Geometry: final body of the model. Coordinates: model frame, mm. Face numbers are marked on the shaded views. A direction names the side the tool comes from. Give positions to 0.01 mm unless a question says otherwise; leave off trailing zeros. Write each loop counter-clockwise with the first axis right and the second up, starting at its lowest first coordinate (ties: lowest second). Pieces come first, ordered by that corner, then holes. Notation, with made-up numbers: M 81.5,-12 L 112.5,-12 A27 ccw 112.5,4 Z; hole C 20.25,36 d2. An arc over 180 degrees is marked long. One line per question, with ' | ' between items.
from build123d import *

# Parameters (mm, degrees)
M3X0_5_TAPPED_HOLE1_D               = 2.5
M3X0_5_TAPPED_HOLE1_DEPTH           = 3.248924226
M3X0_5_TAPPED_HOLE1_TIP             = 0.751075774
BOSS_EXTRUDE1_DEPTH                 = 40
M3X0_5_TAPPED_HOLE2_D               = 2.5
M3X0_5_TAPPED_HOLE2_DEPTH           = 5
M3X0_5_TAPPED_HOLE2_TIP             = 0.751075774
M3X0_5_TAPPED_HOLE2_ON_FACE_2_D     = 2.5
M3X0_5_TAPPED_HOLE2_ON_FACE_2_DEPTH = 5
M3X0_5_TAPPED_HOLE2_ON_FACE_2_TIP   = 0.751075774


with BuildPart() as part:
    # Sketch1 → Revolve1 (revolve)
    with BuildSketch(Plane.XY):
        Polygon((0, 0), (0, 17.5), (10, 17.5), (10, 12.5), (20, 12.5), (20, 17.5), (40, 17.5), (40, 0), align=None)
    revolve(axis=Axis((0, 0, 0), (1, 0, 0)))

    # M3x0.5 Tapped Hole1
    with Locations(Plane(origin=(31.5, 0, 17.5), x_dir=(1, 0, 0), z_dir=(0, 0, 1))):
        with Locations((0, 0)):
            Hole(M3X0_5_TAPPED_HOLE1_D / 2, depth=M3X0_5_TAPPED_HOLE1_DEPTH)
            with Locations((0, 0, -(M3X0_5_TAPPED_HOLE1_DEPTH + M3X0_5_TAPPED_HOLE1_TIP / 2))):  # 118° drill point
                Cone(0, M3X0_5_TAPPED_HOLE1_D / 2, M3X0_5_TAPPED_HOLE1_TIP, mode=Mode.SUBTRACT)

    # Sketch3 → Boss-Extrude1 (add)
    with BuildSketch(Plane(origin=(40, 0, 0), x_dir=(0, 0, -1), z_dir=(1, 0, 0))):
        with BuildLine():
            Line((-12.247448714, -12.5), (-12.247448714, 12.5))
            ThreePointArc((-12.247448714, 12.5), (0, 17.5), (12.247448714, 12.5))
            Line((12.247448714, 12.5), (12.247448714, -12.5))
            ThreePointArc((12.247448714, -12.5), (0, -17.5), (-12.247448714, -12.5))
        make_face()
    extrude(amount=BOSS_EXTRUDE1_DEPTH)

    # M3x0.5 Tapped Hole2
    with Locations(Plane(origin=(50, 0, 12.247448714), x_dir=(1, 0, 0), z_dir=(0, 0, 1))):
        with Locations((0, 0), (15, 0)):
            Hole(M3X0_5_TAPPED_HOLE2_D / 2, depth=M3X0_5_TAPPED_HOLE2_DEPTH)
            with Locations((0, 0, -(M3X0_5_TAPPED_HOLE2_DEPTH + M3X0_5_TAPPED_HOLE2_TIP / 2))):  # 118° drill point
                Cone(0, M3X0_5_TAPPED_HOLE2_D / 2, M3X0_5_TAPPED_HOLE2_TIP, mode=Mode.SUBTRACT)

    # M3x0.5 Tapped Hole2 on face 2
    with Locations(Plane(origin=(65, 0, -12.247448714), x_dir=(-1, 0, 0), z_dir=(0, 0, -1))):
        with Locations((0, 0), (15, 0)):
            Hole(M3X0_5_TAPPED_HOLE2_ON_FACE_2_D / 2, depth=M3X0_5_TAPPED_HOLE2_ON_FACE_2_DEPTH)
            with Locations((0, 0, -(M3X0_5_TAPPED_HOLE2_ON_FACE_2_DEPTH + M3X0_5_TAPPED_HOLE2_ON_FACE_2_TIP / 2))):  # 118° drill point
                Cone(0, M3X0_5_TAPPED_HOLE2_ON_FACE_2_D / 2, M3X0_5_TAPPED_HOLE2_ON_FACE_2_TIP, mode=Mode.SUBTRACT)


solid = part.part
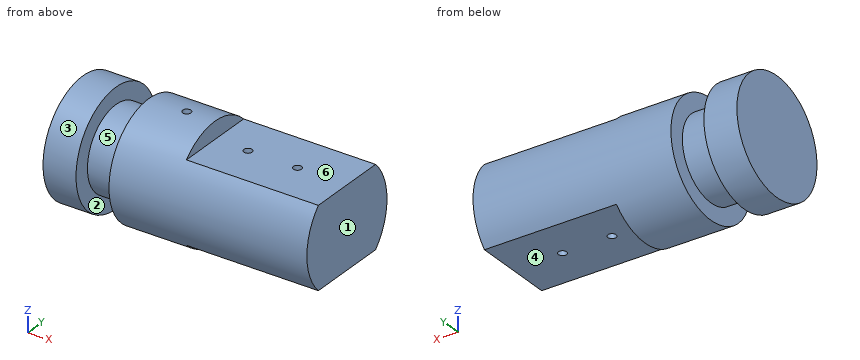
(1) Set-up query: the marked faces 4, 5 and 6. Return all of +Z, -Z, +X, -X, +Y, -Y with unobstructed straight access to the full face (end or side cutting, diameter ignored); none if empty.
Working result:
face 4: -Z, +X, +Y, -Y | face 5: none | face 6: +Z, +X, +Y, -Y
(2) Cut plane A-A, the plane y = -14. Return loops of the section in (x, z), then the cut area to 3 significant figures.
Working result:
outline: M 0,-10.5 L 10,-10.5 L 10,10.5 L 0,10.5 Z; M 20,-10.5 L 80,-10.5 L 80,10.5 L 20,10.5 Z | area: 1,470 mm^2
(3) Cut plane C-C, the plane z = -15. Return loops of the section in (x, y), then the cut area to 3 significant figures.
Working result:
outline: M 0,-9.01 L 10,-9.01 L 10,9.01 L 0,9.01 Z; M 20,-9.01 L 40,-9.01 L 40,9.01 L 20,9.01 Z | area: 541 mm^2
(4) Cut plane D-D, the plane y = -4.5. Return loops of the section in (x, z), then the cut area to 3 significant figures.
Working result:
outline: M 0,-16.91 L 10,-16.91 L 10,-11.66 L 20,-11.66 L 20,-16.91 L 40,-16.91 L 40,-12.25 L 80,-12.25 L 80,12.25 L 40,12.25 L 40,16.91 L 20,16.91 L 20,11.66 L 10,11.66 L 10,16.91 L 0,16.91 Z | area: 2,230 mm^2
(5) Cut plane B-B, the plane z = 0. Return loops of the section in (x, y), then the cut area to 3 significant figures.
Working result:
outline: M 0,-17.5 L 10,-17.5 L 10,-12.5 L 20,-12.5 L 20,-17.5 L 80,-17.5 L 80,17.5 L 20,17.5 L 20,12.5 L 10,12.5 L 10,17.5 L 0,17.5 Z | area: 2,700 mm^2
(6) Material intervals for L1, parallel to X at y = 0, z = -10.7; L2, parallel to X at y = -9, z = -13; L3, parallel to X at y = 9, z = -12, sorted ascending. Write a range as [from, to].
Working result:
L1: x = [0, 48.75], [51.25, 63.75], [66.25, 80] | L2: x = [0, 10], [20, 40] | L3: x = [0, 10], [20, 80]
(7) First-contact query: P1, Ø4, axis at x = 65, y = 0, coming from the +Z side; P2, Ø7.5, axis at x = 65, y = -5.5, coming from the -Z side; P3, Ø1, axis at x = 71, z = 0.5, coming from the +Y side; P4, Ø6, axis at x = 20, z = -4, coming from the -Y side. Flat tips, straight axial feed; report the tip coordinate or a pass-through.
Working result:
P1: stops at z = 12.25 | P2: stops at z = -12.25 | P3: stops at y = 17.5 | P4: stops at y = -17.47
(8) Draft query along X for the marked faces 1, 2 and 3. Return one class per face: released by +X, released by -X, zero draft, split by the parting line, or undercut.
Working result:
face 1: released by +X | face 2: undercut | face 3: zero draft
